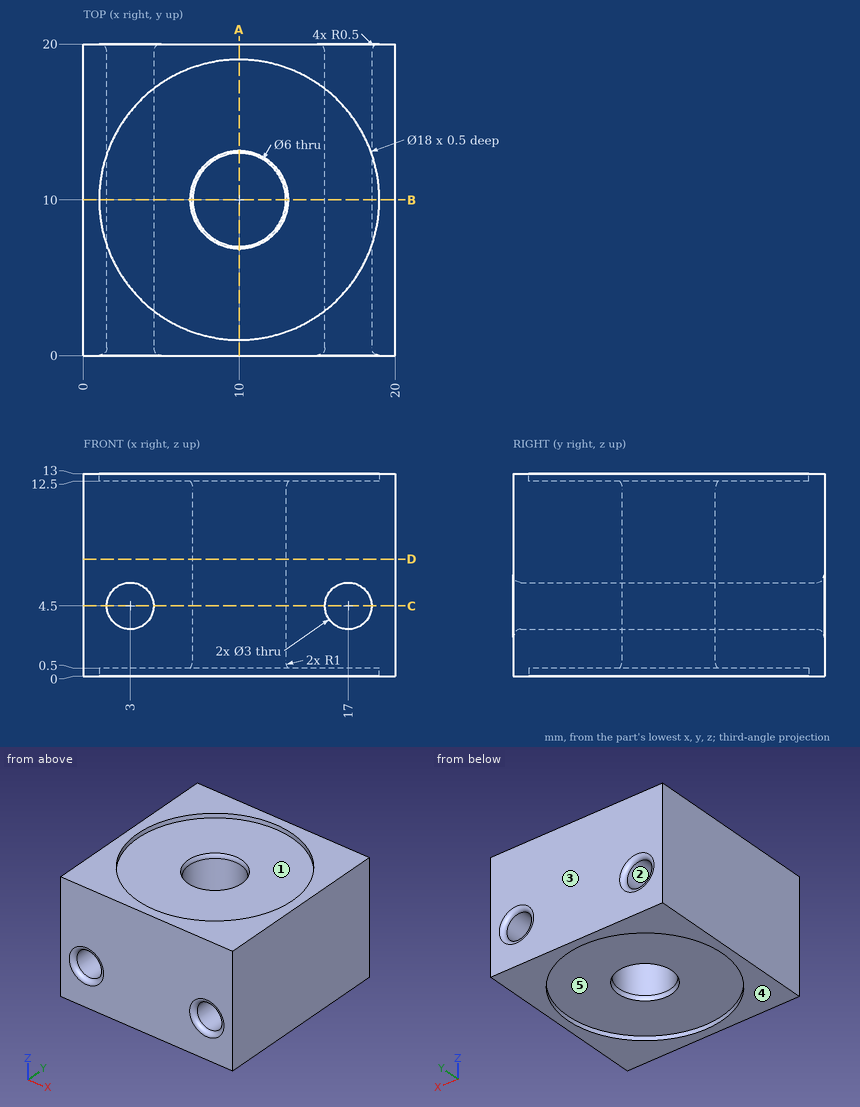
For this review, use the dimensioned drawing (mm, ordinates from the lowest corner) and the shaded views. A direction names the side the tool comes from. Coordinates: 2 decimals unless noted, no trailing zeros. Loops run counter-clockwise (first coordinate to the right, second up) from the corner with the lowest first, then second, coordinate; pieces in that order, holes last. Notation, with made-up numbers: (50, -14.5) - (96, -14.5) arc R26 ccw to (96, 24.5) - close; hole circle Ø5 at (36.25, 39.25). An arc over 180 degrees is marked (long way). Use CSV: the item, a comma, the result in double quotes. Start each with the question number.
1) For pin 1 Ø1.5 at (x, y) = (10.5, 12) entering from -Z; pin 2 Ø11 at (x, y) = (10, 10) entering from -Z; pin 3 Ø5.5 at (x, y) = (11, 13) entering from +Z; pin 4 Ø3.5 at (x, z) = (3, 4.5) entering from -Y, all flat-tipped, find the tip position at first contact; note any pin that passes through.
2) Consider section D-D on z = 7.5. Write out the cut boundary in (x, y), then the cut area to 3 significant figures.
3) Consider section A-A on x = 10. Write out the cut boundary in (y, z).
4) Consider section C-C on z = 4.5. Write out the cut boundary in (x, y).
5) Tool access review of the marked faces 4 and 5: name each direction out of +Z, -Z, +X, -X, +Y, -Y from which nothing blocks a thin tool from reaching the whole face with its end or side.
6) Wall thickness on L1, parallel to Y at x = 10, z = 7.5; L2, parallel to Z at x = 3, y = 7.75; L3, parallel to Y at x = 10, z = 12.7: over which ranges is each line inside the solid? List them lowest first. Write a range as from..to.
7) Consider section B-B on y = 10. Write out the cut boundary in (x, z), then the cut area to 3 significant figures.
8) The part is to be moulded in two halves that separate along Y. For the marked faces 1, 2 and 3, say which applies: +Y half, -Y half, draft (parallel to the pull), parting line (faces both ways), or undercut.
Geometry says:
1,pin 1,"through"
1,pin 2,"z = 0.5"
1,pin 3,"z = 12.5"
1,pin 4,"y = 0.07"
2,outline,"(0, 0) - (20, 0) - (20, 20) - (0, 20) - close; hole circle Ø6 at (10, 10)"
2,area,"372 mm^2"
3,outline,"(0, 0) - (1, 0) - (1, 0.5) - (6.87, 0.5) arc R1 ccw to (7, 1) - (7, 12) arc R1 ccw to (6.87, 12.5) - (1, 12.5) - (1, 13) - (0, 13) - close; (13, 1) arc R1 ccw to (13.13, 0.5) - (19, 0.5) - (19, 0) - (20, 0) - (20, 13) - (19, 13) - (19, 12.5) - (13.13, 12.5) arc R1 ccw to (13, 12) - close"
4,outline,"(0, 0) - (1, 0) arc R0.5 ccw to (1.5, 0.5) - (1.5, 19.5) arc R0.5 ccw to (1, 20) - (0, 20) - close; (4.5, 0.5) arc R0.5 ccw to (5, 0) - (15, 0) arc R0.5 ccw to (15.5, 0.5) - (15.5, 19.5) arc R0.5 ccw to (15, 20) - (5, 20) arc R0.5 ccw to (4.5, 19.5) - close; (18.5, 0.5) arc R0.5 ccw to (19, 0) - (20, 0) - (20, 20) - (19, 20) arc R0.5 ccw to (18.5, 19.5) - close; hole circle Ø6 at (10, 10)"
5,face 4,"-Z, +X, -X, +Y, -Y"
5,face 5,"-Z"
6,L1,"0..7, 13..20"
6,L2,"0.5..3, 6..12.5"
6,L3,"0..1, 19..20"
7,outline,"(0, 0) - (1, 0) - (1, 0.5) - (6.87, 0.5) arc R1 ccw to (7, 1) - (7, 12) arc R1 ccw to (6.87, 12.5) - (1, 12.5) - (1, 13) - (0, 13) - close; (13, 1) arc R1 ccw to (13.13, 0.5) - (19, 0.5) - (19, 0) - (20, 0) - (20, 13) - (19, 13) - (19, 12.5) - (13.13, 12.5) arc R1 ccw to (13, 12) - close; hole circle Ø3 at (3, 4.5); hole circle Ø3 at (17, 4.5)"
7,area,"156 mm^2"
8,face 1,"undercut"
8,face 2,"draft"
8,face 3,"+Y half"
